Geometry check sheet. Reference: drawing and pictorial views, mm from the part's lowest x, y, z. A direction names the side the tool comes from. Round coordinates to 2 decimals unless told otherwise and drop trailing zeros. Order: outer loops, then holes, each group sorted by start corner. A loop starts at its lowest first (then second) coordinate and runs counter-clockwise, first axis right, second up.
(1) Release check for a two-part mould opening along Y. For the marked faces 1, 2 and 3 record: +Y half, -Y half, draft (parallel to the pull), parting line (faces both ways), or undercut.
(2) Sectioned sample at D-D (x = 15.75). Record the boundary of the cut face in (y, z), plus the area to 3 significant figures.
(3) Go/stop test with flat-tipped pins: pin 1 (2 mm diameter, centred on x = 11, z = 9.5, fed in from -Y); pin 2 (6 mm diameter, centred on x = 4, z = 7.5, fed in from +Y); pin 3 (1.5 mm diameter, centred on y = 4, z = 7.5, fed in from +X). Record where each tip stops, or that it passes through.
(4) Sectioned sample at A-A (x = 8.5). Record the boundary of the cut face in (y, z), plus the area to 3 significant figures.
(5) Material ranges on line 1 along Z through (x, y) = (15.5, 8.25); line 2 along Y through (x, z) = (8.5, 13.5); line 3 along Z through (x, y) = (13.25, 4.5), recorded low to high.
(6) Sectioned sample at C-C (z = 3.5). Record the boundary of the cut face in (x, y), plus the area to 3 significant figures.
(7) Set-up check for the marked faces 4, 5 and 6: record each of +Z, -Z, +X, -X, +Y, -Y from which the full face is reachable in a straight line by a thin tool's end or side.
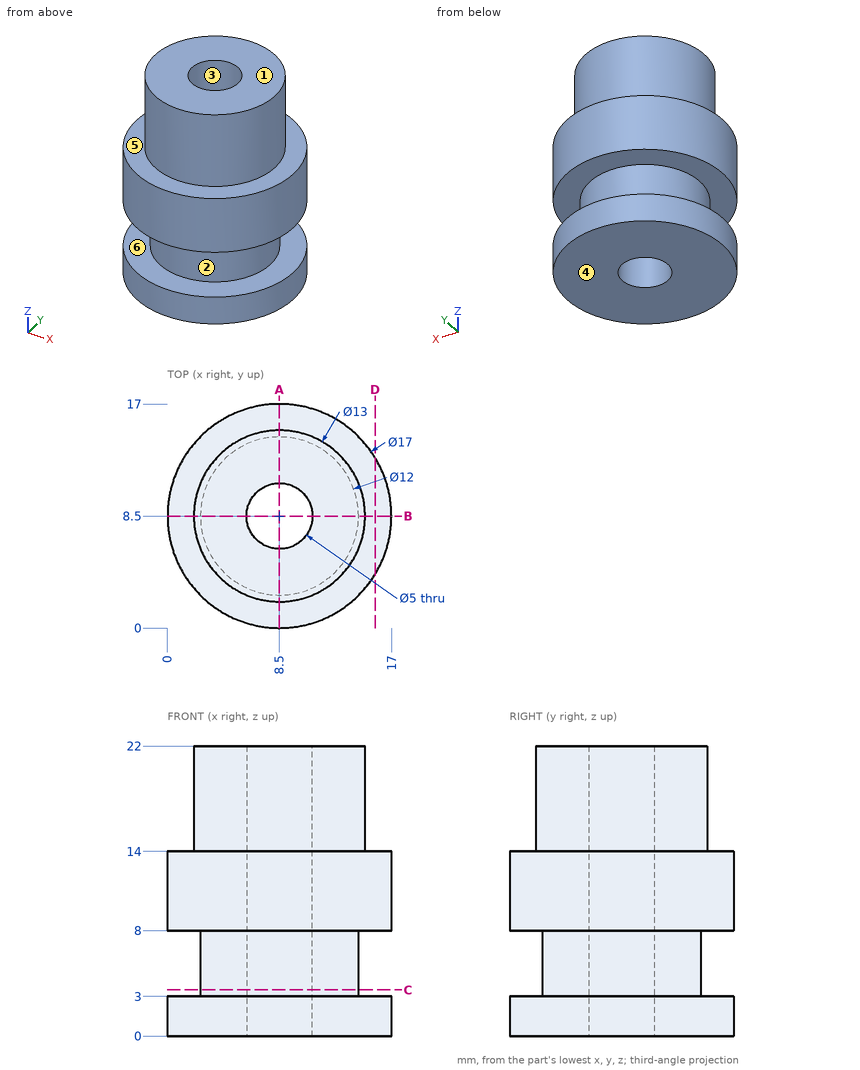
Answer below:
1. face 1: draft
1. face 2: parting line
1. face 3: undercut
2. outline: (4.06, 0) - (12.94, 0) - (12.94, 3) - (4.06, 3) - close; (4.06, 8) - (12.94, 8) - (12.94, 14) - (4.06, 14) - close
2. area: 79.9 mm2
3. pin 1: stops at y = 0.13
3. pin 2: stops at y = 16.86
3. pin 3: stops at x = 16.03
4. outline: (0, 0) - (6, 0) - (6, 22) - (2, 22) - (2, 14) - (0, 14) - (0, 8) - (2.5, 8) - (2.5, 3) - (0, 3) - close; (11, 0) - (17, 0) - (17, 3) - (14.5, 3) - (14.5, 8) - (17, 8) - (17, 14) - (15, 14) - (15, 22) - (11, 22) - close
4. area: 207 mm2
5. line 1: z = 0 to 3, 8 to 14
5. line 2: y = 0 to 6, 11 to 17
5. line 3: z = 0 to 3, 8 to 22
6. outline: circle Ø12 at (8.5, 8.5); hole circle Ø5 at (8.5, 8.5)
6. area: 93.5 mm2
7. face 4: -Z, +X, -X, +Y, -Y
7. face 5: +Z
7. face 6: none
